Could you check a few things on this drawing? It's one solid part, dimensions in mm from its lowest x, y, z. A direction names the side the tool comes from. Coordinates: 2 decimals unless noted, no trailing zeros. Order: outer loops, then holes, each group sorted by start corner. A loop starts at its lowest first (then second) coordinate and runs counter-clockwise, first axis right, second up.
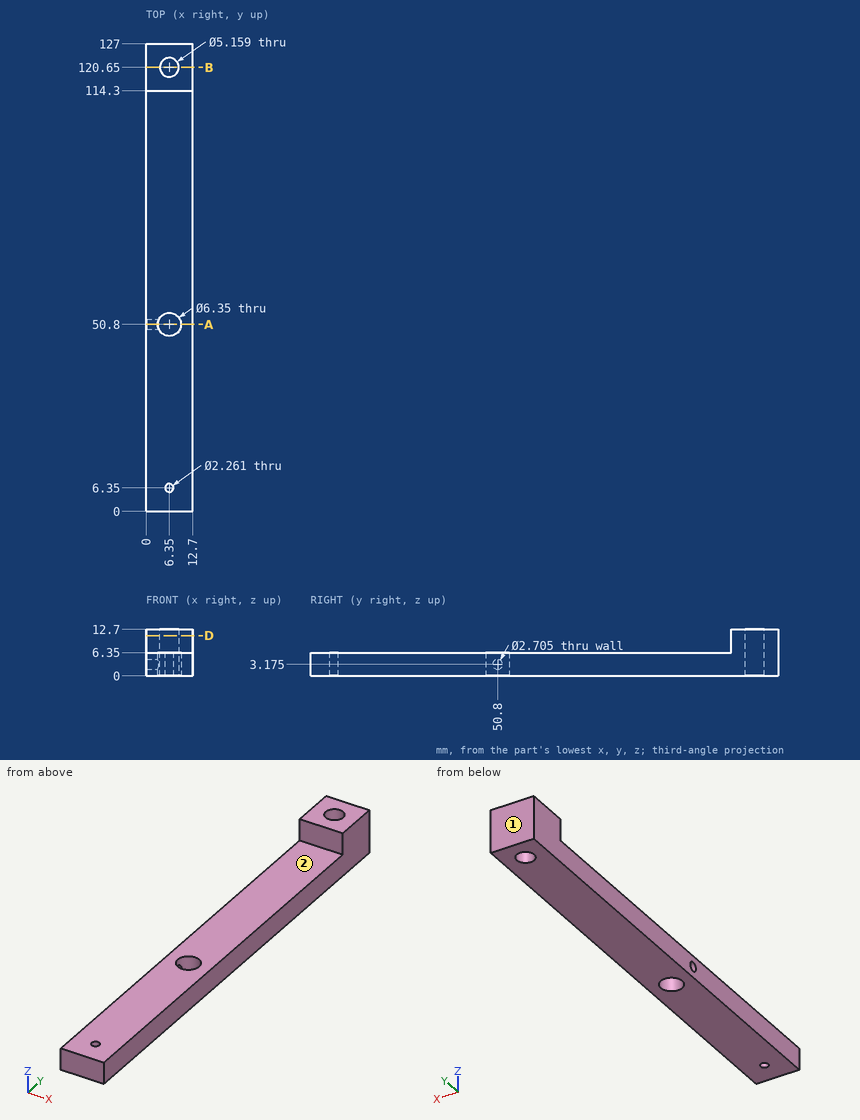
Q1. If we section it at D-D on z = 11: Write out the boundary of the cut face in (x, y).
Q2. For the marked faces 1 and 2, which set-ups out of +Z, -Z, +X, -X, +Y, -Y let a thin tool reach every point of the face, with its end or its side?
Q3. If we section it at B-B on y = 120.65: Write out the boundary of the cut face in (x, z).
Q4. I need wall thicknesses on L1, parallel to Y at x = 6.35, z = 3 (1 decimal); L2, parallel to Z at x = 1.3, y = 50.8; L3, parallel to Y at x = 6.35, z = 6.75. Which ranges of each line are inside material? Lowest first, please.
Q5. If we section it at A-A on y = 50.8: Give the number of separate pieces and of enclosed holes in the cut face.
Q6. Will these pins go through, and if not, where does the flat tip stop? pin 1 (5 mm diameter, centred on x = 7, y = 18.5, fed in from +Z); pin 2 (4.5 mm diameter, centred on x = 6.35, y = 120.65, fed in from +Z); pin 3 (1.9 mm diameter, centred on x = 4.5, z = 11, fed in from -Y).
Reply:
1. outline: (0, 114.3) - (12.7, 114.3) - (12.7, 127) - (0, 127) - close; hole circle Ø5.16 at (6.35, 120.65)
2. face 1: +Z, -Z, +X, -X, +Y
2. face 2: +Z, +X, -X, -Y
3. outline: (0, 0) - (3.77, 0) - (3.77, 12.7) - (0, 12.7) - close; (8.93, 0) - (12.7, 0) - (12.7, 12.7) - (8.93, 12.7) - close
4. L1: y = 0 to 5.2, 7.5 to 47.6, 54 to 118.1, 123.2 to 127
4. L2: z = 0 to 1.82, 4.53 to 6.35
4. L3: y = 114.3 to 118.07, 123.23 to 127
5. separate pieces: 3
5. enclosed holes: 0
6. pin 1: stops at z = 6.35
6. pin 2: passes through
6. pin 3: stops at y = 114.3
